Here's the drawing with two shaded views (mm, measured from the low corner). I have some questions. A direction names the side the tool comes from. Give positions to 0.01 mm unless a question says otherwise; leave off trailing zeros. Loops run counter-clockwise (first coordinate to the right, second up) from the corner with the lowest first, then second, coordinate; pieces in that order, holes last.
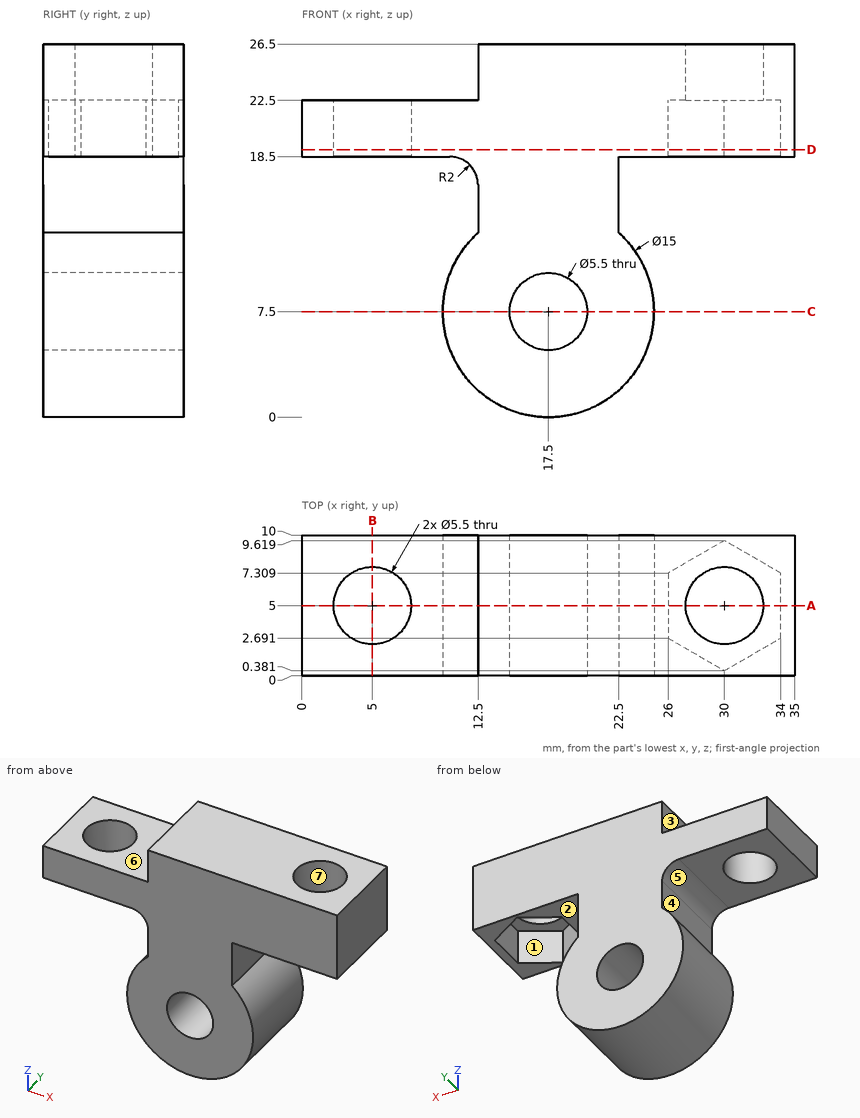
(1) Will these pins go through, and if not, where does the flat tip stop? P1, Ø1, axis at x = 10, y = 8.5, coming from the +Z side; P2, Ø6, axis at y = 1, z = 6, coming from the -X side; P3, Ø1.6, axis at y = 5.5, z = 15, coming from the +X side.
Returned:
P1: stops at z = 22.5
P2: stops at x = 10
P3: stops at x = 22.5
(2) Please list where these lines run through material, in increasing order: probe 1 along X at (y, z) = (4, 20.75); probe 2 along Y at (x, z) = (30, 24.45); probe 3 along Z at (x, y) = (17.5, 6).
Returned:
probe 1: x = 0 to 2.44, 7.56 to 26, 34 to 35
probe 2: y = 0 to 2.25, 7.75 to 10
probe 3: z = 0 to 4.75, 10.25 to 26.5
(3) Suppose I cut it at D-D on z = 19. List the corners of the cut face in (x, y) for me, plus the area to 3 significant figures.
Returned:
outline: (0, 0) - (35, 0) - (35, 10) - (0, 10) - close; hole circle Ø5.5 at (5, 5); hole (26, 2.69) - (30, 0.38) - (34, 2.69) - (34, 7.31) - (30, 9.62) - (26, 7.31) - close
area: 271 mm2
(4) Suppose I cut it at A-A on y = 5. List the corners of the cut face in (x, z) for me, plus the area to 3 significant figures.
Returned:
outline: (0, 18.5) - (2.25, 18.5) - (2.25, 22.5) - (0, 22.5) - close; (7.75, 18.5) - (10.5, 18.5) arc R2 cw to (12.5, 16.5) - (12.5, 13.09) arc R7.5 ccw (long way) to (22.5, 13.09) - (22.5, 18.5) - (26, 18.5) - (26, 22.5) - (27.25, 22.5) - (27.25, 26.5) - (12.5, 26.5) - (12.5, 22.5) - (7.75, 22.5) - close; (32.75, 22.5) - (34, 22.5) - (34, 18.5) - (35, 18.5) - (35, 26.5) - (32.75, 26.5) - close; hole circle Ø5.5 at (17.5, 7.5)
area: 349 mm2
(5) Suppose I cut it at C-C on z = 7.5. List the corners of the cut face in (x, y) for me.
Returned:
outline: (10, 0) - (14.75, 0) - (14.75, 10) - (10, 10) - close; (20.25, 0) - (25, 0) - (25, 10) - (20.25, 10) - close
(6) Which directions (+Z, -Z, +X, -X, +Y, -Y) give clear straight access to the entire face, cutting with the end or side of a thin tool? Please do the marked faces 1, 2, 3 and 4.
Returned:
face 1: -Z
face 2: +X, +Y, -Y
face 3: +Z, -X, +Y, -Y
face 4: -X, +Y, -Y
(7) Suppose I cut it at B-B on x = 5. List the corners of the cut face in (y, z) for me, plus the area to 3 significant figures.
Returned:
outline: (0, 18.5) - (2.25, 18.5) - (2.25, 22.5) - (0, 22.5) - close; (7.75, 18.5) - (10, 18.5) - (10, 22.5) - (7.75, 22.5) - close
area: 18.0 mm2
(8) Thinking about a two-plate mould opening in Z: for the marked faces 5, 6 and 7, which applies, pulls with the +Z half, pulls with the -Z half, needs draft (parallel to the pull), parting line crosses it, or undercut?
Returned:
face 5: undercut
face 6: pulls with the +Z half
face 7: needs draft
